Design review of the part built by this model. Coordinates are the model's own, in mm. Coordinates: 2 decimals unless noted, no trailing zeros. Write each loop counter-clockwise with the first axis right and the second up, starting at its lowest first coordinate (ties: lowest second). Pieces come first, ordered by that corner, then holes. Notation, with made-up numbers: (66.25, 55.5) - (72.25, 55.5) arc R30 cw to (72.25, 85.5) - close; hole circle Ø4 at (2.5, 2.25). An arc over 180 degrees is marked (long way). One line per item, written item: value.
from build123d import *

# Parameters (mm, degrees)
F3_DEPTH = 6
F4_DEPTH = 1


# Not quite as in the source:
# - a feature of the source that left no trace in its solid (it failed there, or was rolled back) is left out


with BuildPart() as f3:
    # F0 (on Top) → F3 (new body)
    with BuildSketch(Plane.XY):
        with BuildLine():
            ThreePointArc((0, 1.25), (0.8838834765, 0.8838834765), (1.25, 0))
            Line((1.25, 0), (10, 0))
            ThreePointArc((10, 0), (7.0710678119, 7.0710678119), (0, 10))
            Line((0, 10), (0, 1.25))
        make_face()
        with BuildLine():
            ThreePointArc((0, 0.5), (0.3535533906, 0.3535533906), (0.5, 0))
            Line((0.5, 0), (1.25, 0))
            ThreePointArc((1.25, 0), (0.8838834765, 0.8838834765), (0, 1.25))
            Line((0, 1.25), (0, 0.5))
        make_face()
        with BuildLine():
            Line((0, 0), (0.5, 0))
            ThreePointArc((0.5, 0), (0.3535533906, 0.3535533906), (0, 0.5))
            Line((0, 0.5), (0, 0))
        make_face()
    extrude(amount=-F3_DEPTH)

    # F0 (on Top) → F4 (cut)
    with BuildSketch(Plane.XY):
        with BuildLine():
            Line((0, 0), (0.5, 0))
            ThreePointArc((0.5, 0), (0.3535533906, 0.3535533906), (0, 0.5))
            Line((0, 0.5), (0, 0))
        make_face()
    extrude(amount=-F4_DEPTH, mode=Mode.SUBTRACT)


solid = f3.part
1. Wall thickness on line 1 along Y through (x, z) = (5.25, -0.7); line 2 along Y through (x, z) = (6.25, -2.55): over which ranges is each line inside the solid? List them lowest first.
Answer block:
line 1: y = 0 to 8.51
line 2: y = 0 to 7.81
2. Consider section A-A, the plane z = -5.2. Write out the cut boundary in (x, y), then the cut area to 3 significant figures.
Answer block:
outline: (0, 0) - (10, 0) arc R10 ccw to (0, 10) - close
area: 78.5 mm^2
3. Consider section B-B, the plane y = 6. Write out the cut boundary in (x, z).
Answer block:
outline: (0, -6) - (8, -6) - (8, 0) - (0, 0) - close
4. Consider section C-C, the plane x = 5.5. Write out the cut boundary in (y, z), then the cut area to 3 significant figures.
Answer block:
outline: (0, -6) - (8.35, -6) - (8.35, 0) - (0, 0) - close
area: 50.1 mm^2
5. Insertion check: pin 1 Ø1.5 at (y, z) = (1.5, -5) entering from +X. The pin has a flat end and moves straight along its axis. Give the tip position at first contact, or say it passes through.
Answer block:
pin 1: stops at x = 9.97
